from build123d import *

# Parameters (mm, degrees)
F1_DEPTH = 15


with BuildPart() as f1:
    # F0 (on Right) → F1 (new body)
    with BuildSketch(Plane.YZ):
        with BuildLine():
            ThreePointArc((35, 14.5), (32.656854, 20.156854), (27, 22.5))
            Line((27, 22.5), (-27, 22.5))
            ThreePointArc((-27, 22.5), (-32.656854, 20.156854), (-35, 14.5))
            Line((-35, 14.5), (-35, 6.617025))
            Line((-35, 6.617025), (-20, 6.617025))
            Line((-20, 6.617025), (-20, -8.382975))
            Line((-20, -8.382975), (-35, -8.382975))
            Line((-35, -8.382975), (-35, -14.5))
            ThreePointArc((-35, -14.5), (-32.656854, -20.156854), (-27, -22.5))
            Line((-27, -22.5), (27, -22.5))
            ThreePointArc((27, -22.5), (32.656854, -20.156854), (35, -14.5))
            Line((35, -14.5), (35, -8.382975))
            Line((35, -8.382975), (20, -8.382975))
            Line((20, -8.382975), (20, 6.617025))
            Line((20, 6.617025), (35, 6.617025))
            Line((35, 6.617025), (35, 14.5))
        make_face()
    extrude(amount=F1_DEPTH)


solid = f1.part
Geometry: final body of the model. Coordinates: model frame, mm. A direction names the side the tool comes from. Round coordinates to 2 decimals unless told otherwise and drop trailing zeros. Loops run counter-clockwise (first coordinate to the right, second up) from the corner with the lowest first, then second, coordinate; pieces in that order, holes last. Notation, with made-up numbers: (-7, -12.5) - (21, -12.5) arc R7 cw to (21, -1.5) - close; hole circle Ø2 at (86.25, -22.5). An arc over 180 degrees is marked (long way). Write each question's results on one line, items separated by ' | '. Start each with the question number.
1) First-contact query: P1, Ø3, axis at x = 12, z = 1, coming from the -Y side. Flat tip, straight axial feed; report the tip coordinate or a pass-through.
2) Cut plane A-A on y = -23. Return loops of the section in (x, z), then the cut area to 3 significant figures.
3) Cut plane B-B on x = 12. Return loops of the section in (y, z).
4) Mould query, pull axis Z, two halves, no side actions, for faces 4 (the face through (7, 27, 6.617)), 5 (the face through (7.395, -32.719, -20.094)), 6 (the face through (7, 35, 11)). Classes: released by +Z, released by -Z, zero draft, split by the parting line, or undercut.
5) Access query for faces 1 (the face through (7, -20, -1)), 2 (the face through (7, 20, -1)), 3 (the face through (7, 0, 22.5)). Directions: +Z, -Z, +X, -X, +Y, -Y. A direction counts if a zero-diameter tool reaches every point of the face in a straight line with its end or side. Return the directions, or none.
6) Line query: probe 1 along Z at (x, y) = (1, 26); probe 2 along Y at (x, z) = (8, 6); probe 3 along Z at (x, y) = (5, -31). Output: solid intervals per line, ascending. Write a range as [from, to].
7) Cut plane D-D on z = 19. Return loops of the section in (x, y).
8) Cut plane C-C on z = 4. Return loops of the section in (x, y).
Verdict:
1) P1: stops at y = -20
2) outline: (0, -22.5) - (15, -22.5) - (15, -8.38) - (0, -8.38) - close; (0, 6.62) - (15, 6.62) - (15, 22.5) - (0, 22.5) - close | area: 450 mm2
3) outline: (-35, -14.5) arc R8 ccw to (-27, -22.5) - (27, -22.5) arc R8 ccw to (35, -14.5) - (35, -8.38) - (20, -8.38) - (20, 6.62) - (35, 6.62) - (35, 14.5) arc R8 ccw to (27, 22.5) - (-27, 22.5) arc R8 ccw to (-35, 14.5) - (-35, 6.62) - (-20, 6.62) - (-20, -8.38) - (-35, -8.38) - close
4) face 4: undercut | face 5: released by -Z | face 6: zero draft
5) face 1: +X, -X, -Y | face 2: +X, -X, +Y | face 3: +Z, +X, -X, +Y, -Y
6) probe 1: z = [-22.5, -8.38], [6.62, 22.5] | probe 2: y = [-20, 20] | probe 3: z = [-21.43, -8.38], [6.62, 21.43]
7) outline: (0, -33.61) - (15, -33.61) - (15, 33.61) - (0, 33.61) - close
8) outline: (0, -20) - (15, -20) - (15, 20) - (0, 20) - close
